Could you check a few things on this drawing? It's one solid part, dimensions in mm from its lowest x, y, z. Give positions to 0.01 mm unless a question says otherwise; leave off trailing zeros. Loops run counter-clockwise (first coordinate to the right, second up) from the corner with the lowest first, then second, coordinate; pieces in that order, holes last. Notation, with made-up numbers: (-12, 13) -> (8, 13) arc R18 cw to (8, 34) -> close; hole circle Ø10 at (-17.75, 87). An arc over 180 degrees is marked (long way). Use CSV: the item, a comma, the result in double quotes.
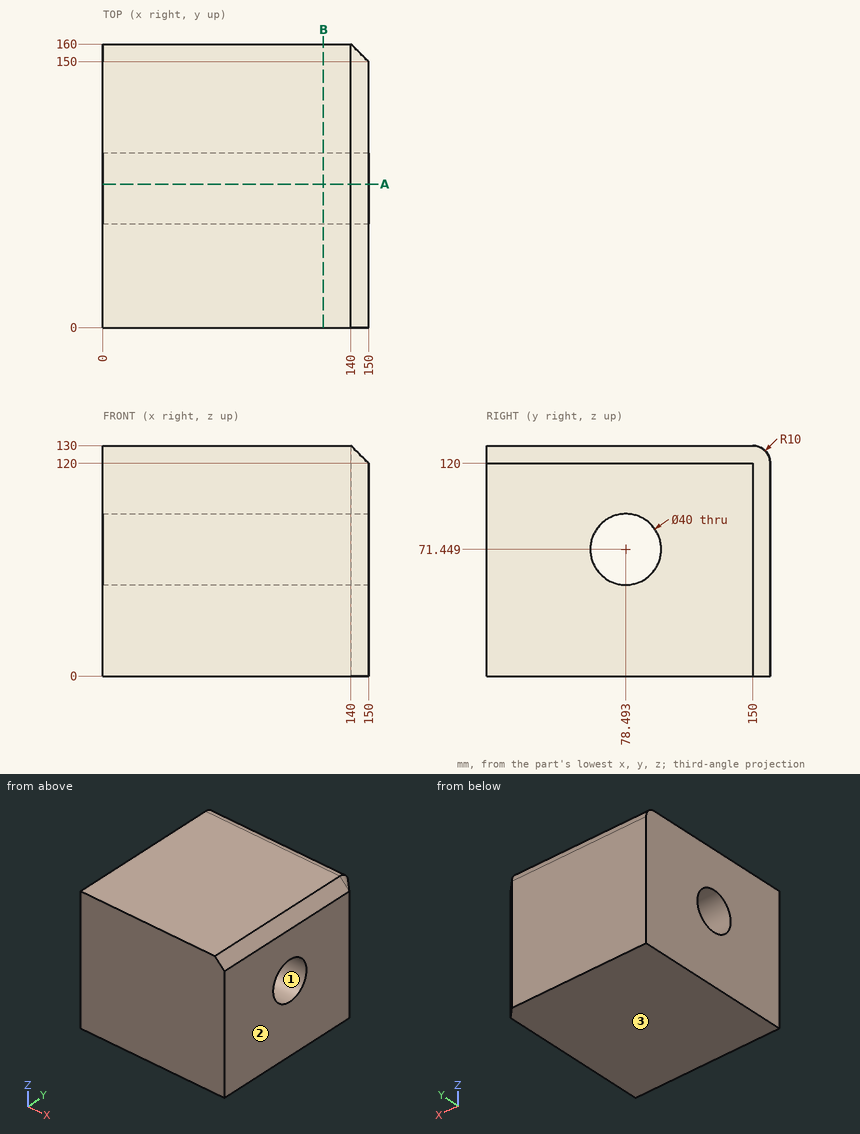
(1) If we section it at B-B, the plane x = 124.5: Write out the boundary of the cut face in (y, z).
Answer sheet:
outline,"(0, 0) -> (160, 0) -> (160, 120) arc R10 ccw to (150, 130) -> (0, 130) -> close; hole circle Ø40 at (78.49, 71.45)"
(2) If I drill on L1, parallel to Z at x = 121, y = 75; L2, parallel to Z at x = 121, y = 86; L3, parallel to Y at x = 77.5, z = 85, over which ranges is the centre line in solid material (lowest first)? Write a range as from..to.
Answer sheet:
L1,"z = 0..51.76, 91.14..130"
L2,"z = 0..52.91, 89.99..130"
L3,"y = 0..63.78, 93.2..160"
(3) We'd pull the mould along Z, two halves only. Please class the marked faces 1, 2 and 3: released by +Z, released by -Z, zero draft, split by the parting line, or undercut.
Answer sheet:
face 1,"undercut"
face 2,"zero draft"
face 3,"released by -Z"
(4) If we section it at A-A, the plane y = 81: Write out the boundary of the cut face in (x, z), then the cut area to 3 significant figures.
Answer sheet:
outline,"(0, 0) -> (150, 0) -> (150, 51.61) -> (0, 51.61) -> close; (0, 91.29) -> (150, 91.29) -> (150, 120) -> (140, 130) -> (0, 130) -> close"
area,"13,500 mm2"
